Can you work these out from the model? Positions are in its coordinate system, mm. A direction names the side the tool comes from. Give positions to 0.01 mm unless a question says otherwise; leave off trailing zeros. Write each loop counter-clockwise with the first axis right and the second up, starting at its lowest first coordinate (ties: lowest second). Pieces come first, ordered by that corner, then holes. Notation, with made-up numbers: (-20.75, -25.75) - (-3.75, -25.75) arc R18 ccw to (-3.75, -7.75) - close; hole circle Ø6 at (87.5, -21.75). An arc over 180 degrees is marked (long way). Use a Markdown table: item, result. Add a question column.
```python
from build123d import *

# Parameters (mm, degrees)
SKETCH1_R           = 65.151
SKETCH1_R_2         = 42.926
BOSS_EXTRUDE2_DEPTH = 7.874
SKETCH1_5_R         = 73.025
SKETCH1_5_R_2       = 65.151
BOSS_EXTRUDE3_DEPTH = 38.1
SKETCH24_R          = 5.588
CUT_EXTRUDE1_DEPTH  = 38.1
CIRPATTERN3_COUNT   = 8
BOSS_EXTRUDE7_START = -7.874
BOSS_EXTRUDE7_DEPTH = 7.874
SKETCH35_R          = 5.588
CUT_EXTRUDE2_DEPTH  = 111.076842611
CIRPATTERN9_COUNT   = 4


with BuildPart() as part:
    # Sketch1 → Boss-Extrude2 (new body)
    with BuildSketch(Plane(origin=(0, 0, 0), x_dir=(0, 0, -1), z_dir=(1, 0, 0))):
        Circle(SKETCH1_R)
        Circle(SKETCH1_R_2, mode=Mode.SUBTRACT)
    extrude(amount=BOSS_EXTRUDE2_DEPTH)

    # Sketch1_5 → Boss-Extrude3 (add)
    with BuildSketch(Plane(origin=(0, 0, 0), x_dir=(0, 0, -1), z_dir=(1, 0, 0))):
        with Locations(Location((0, 0, 0), (0, 0, 180))):
            Circle(SKETCH1_5_R)
        with Locations(Location((0, 0, 0), (0, 0, 180))):
            Circle(SKETCH1_5_R_2, mode=Mode.SUBTRACT)
    extrude(amount=BOSS_EXTRUDE3_DEPTH)

    # Sketch24 → Cut-Extrude1 (cut)
    with BuildSketch(Plane(origin=(7.874, 0, 0), x_dir=(0, 0, -1), z_dir=(1, 0, 0))):
        with Locations((0, 54.991)):
            Circle(SKETCH24_R)
    cut_extrude1 = extrude(amount=-CUT_EXTRUDE1_DEPTH, mode=Mode.SUBTRACT)

    # CirPattern3: Cut-Extrude1 ×8 about axis
    cirpattern3_axis = Axis((0, 0, 0), (1, 0, 0))
    for i in range(1, CIRPATTERN3_COUNT):
        add(cut_extrude1.rotate(cirpattern3_axis, i * 360 / CIRPATTERN3_COUNT), mode=Mode.SUBTRACT)

    # Sketch34 → Boss-Extrude7 (add)
    with BuildSketch(Plane(origin=(38.1, 0, 0), x_dir=(0, 0, -1), z_dir=(1, 0, 0)).offset(BOSS_EXTRUDE7_START)):
        with BuildLine():
            Line((10.881292196, -53.903687825), (10.881292196, -64.235895581))
            ThreePointArc((10.881292196, -64.235895581), (0, -65.151), (-10.881292196, -64.235895581))
            Line((-10.881292196, -64.235895581), (-10.881292196, -53.903687825))
            add(Edge.make_bspline(
                [(10.881292196, -53.903687825), (9.981727061, -42.926), (0, -42.926), (-9.981727061, -42.926), (-10.881292196, -53.903687825)],
                knots=[1.661039958, 1.661039958, 1.661039958, 3.141592654, 3.141592654, 4.622145349, 4.622145349, 4.622145349], degree=2, weights=[1, 0.738282192, 1, 0.738282192, 1]))
        make_face()
    boss_extrude7 = extrude(amount=BOSS_EXTRUDE7_DEPTH)

    # Sketch35 → Cut-Extrude2 (cut, through all)
    with BuildSketch(Plane(origin=(38.1, 0, 0), x_dir=(0, 0, -1), z_dir=(1, 0, 0))):
        with Locations(Location((0, -54.991, 0), (0, 0, 180))):
            Circle(SKETCH35_R)
    cut_extrude2 = extrude(amount=-CUT_EXTRUDE2_DEPTH, mode=Mode.SUBTRACT)

    # CirPattern9: Boss-Extrude7, Cut-Extrude2 ×4 about axis
    cirpattern9_axis = Axis((38.1, 0, 0), (-1, 0, 0))
    add([boss_extrude7.rotate(cirpattern9_axis, i * 360 / CIRPATTERN9_COUNT) for i in range(1, CIRPATTERN9_COUNT)])
    add([cut_extrude2.rotate(cirpattern9_axis, i * 360 / CIRPATTERN9_COUNT) for i in range(1, CIRPATTERN9_COUNT)], mode=Mode.SUBTRACT)


solid = part.part
```
Q1. Suppose I cut it at A-A (z = -25). Please give me the cut outline in (x, y).
Q2. If I drill on probe 1 along Y at (x, z) = (36, 0) (3 decimals); probe 2 along Z at (x, y) = (32, 56); probe 3 along Y at (x, z) = (35.5, 46), over which ranges is the centre line in solid material (lowest first)? Write a range as [from, to].
Q3. If we mould it in two halves opening along Y, with no side actions, what happens to faces 1 (the cylindrical face through (18.783, 64.786, 33.697)), 2 (the flat face through (0, 31, 31)), 3 (the flat face through (34, -10.881, -59))? For each: released by +Y, released by -Y, zero draft, split by the parting line, or undercut.
Q4. Suppose I cut it at D-D (y = 0). Give the number of separate pieces and of enclosed holes in the cut face, and give its area (3 significant figures).
Q5. Suppose I cut it at B-B (x = 19). Please give me the cut outline in (y, z) (3 decimals), and give its area (3 significant figures).
Q6. On a 3-axis mill with a long thin cutter (end or side, diameter ignored), from which of +Z, -Z, +X, -X, +Y, -Y can I reach the whole of each face in a straight line? I mean faces 4 (the flat face through (34, -59, 10.881)), 5 (the cylindrical face through (3.882, 12.894, -40.944)), 6 (the flat face through (30.226, 51, -5)). Say none if no direction works.
Q7. Suppose I cut it at C-C (z = 37). Please give me the cut outline in (x, y), and give its area (3 significant figures).
Q8. I'm going to push flat-ended pins straight in: P1, Ø4, axis at x = 34, z = -59.5, coming from the -Y side; P2, Ø12, axis at x = 25.5, z = -28.5, coming from the +Y side; P3, Ø8.5, axis at x = 32, z = 59, coming from the +Y side; P4, Ø9, axis at y = 0, z = -54.991, coming from the -X side. Where does each tip first touch, or does it pass through?
Derived:
| question | item | result |
|---|---|---|
| 1 | outline | (0, -68.61) - (38.1, -68.61) - (38.1, -60.16) - (7.87, -60.16) - (7.87, -34.89) - (0, -34.89) - close; (0, 34.89) - (7.87, 34.89) - (7.87, 60.16) - (38.1, 60.16) - (38.1, 68.61) - (0, 68.61) - close |
| 2 | probe 1 | [-73.025, -60.579], [-49.403, -42.926], [42.926, 49.403], [60.579, 73.025] |
| 2 | probe 2 | [-46.87, -33.3], [-10.88, -5.5], [5.5, 10.88], [33.3, 46.87] |
| 2 | probe 3 | [-56.72, -46.14], [-7.29, 7.29], [46.14, 56.72] |
| 3 | face 1 | split by the parting line |
| 3 | face 2 | zero draft |
| 3 | face 3 | undercut |
| 4 | separate pieces | 6 |
| 4 | enclosed holes | 0 |
| 4 | area | 948 mm² |
| 5 | outline | circle Ø146.05 at (0, 0); hole circle Ø130.302 at (0, 0) |
| 5 | area | 3,420 mm² |
| 6 | face 4 | +X |
| 6 | face 5 | +X, -X |
| 6 | face 6 | none |
| 7 | outline | (0, -62.96) - (38.1, -62.96) - (38.1, -53.63) - (7.87, -53.63) - (7.87, -44.15) - (0, -44.15) - close; (0, -33.62) - (7.87, -33.62) - (7.87, -21.76) - (0, -21.76) - close; (0, 21.76) - (7.87, 21.76) - (7.87, 33.62) - (0, 33.62) - close; (0, 44.15) - (7.87, 44.15) - (7.87, 53.63) - (38.1, 53.63) - (38.1, 62.96) - (0, 62.96) - close |
| 7 | area | 1,050 mm² |
| 8 | P1 | y = -45.02 |
| 8 | P2 | y = 69.47 |
| 8 | P3 | y = 48.32 |
| 8 | P4 | through |
